For this review, take the finished solid that the model builds, in its own axes (mm). A direction names the side the tool comes from. Coordinates: 2 decimals unless noted, no trailing zeros. Loops run counter-clockwise (first coordinate to the right, second up) from the corner with the lowest first, then second, coordinate; pieces in that order, holes last. Notation, with made-up numbers: (78, 83) -> (83, 83) arc R25 ccw to (83, 101) -> close; hole circle Ø10 at (-38, 80). An arc over 180 degrees is marked (long way). Use a Markdown table: item, result.
from build123d import *

# Parameters (mm, degrees)
SKETCH1_W                           = 18.5
SKETCH1_H                           = 19.8
BE_00_BODY_DEPTH                    = 5.3
CE_00_MAIN_CAVITY_DEPTH             = 0.7112
CUT_EXTRUDE26_DEPTH                 = 1.5
CE_00_OUTPUT_CAVITY_DEPTH           = 2.75
CE_00_MULTIPIN_CAVITY_DEPTH         = 3.66
SKETCH43_W                          = 24.756879044
SKETCH43_H                          = 5.996687822
CE_00_NEAR_MULTIPIN_CONNECTOR_DEPTH = 2.75
CE_00_DC_BOARD_CAVITY_DEPTH         = 2
FILLET_A_0_4MM_R                    = 0.4
FILLET_B_0_2_R                      = 0.2
FILLET_C_0_16MM_R                   = 0.16
FILLET_E_0_05MM_R                   = 0.05
CHAMFER_A_0_10MM_SIZE               = 0.1
CHAMFER1_SIZE                       = 0.0508


# Read off the part's stored shape, not the designer's step: CSK for #0 Flat Head Machine Screw2
with BuildPart() as part:
    # Sketch1 → BE-00 Body (new body)
    with BuildSketch(Plane(origin=(0, 0, 0), x_dir=(1, 0, 0), z_dir=(0, 1, 0))):
        with Locations((0.75, 3.1)):
            Rectangle(SKETCH1_W, SKETCH1_H)
    extrude(amount=BE_00_BODY_DEPTH)

    # Sketch9 → CE-00 Main Cavity (cut)
    with BuildSketch(Plane(origin=(0, 0, 0), x_dir=(1, 0, 0), z_dir=(0, 1, 0))):
        with BuildLine():
            Line((2.146781775, -1.5534), (12.535922666, -1.5534))
            Line((12.535922666, -1.5534), (12.535922666, 2.0534))
            Line((12.535922666, 2.0534), (2.2, 2.0534))
            Line((2.2, 2.0534), (2.2, 6.384290248))
            Line((2.2, 6.384290248), (0, 6.384290248))
            Line((0, 6.384290248), (0, 2.4))
            Line((0, 2.4), (-10.40064316, 2.4))
            Line((-10.40064316, 2.4), (-10.40064316, -2.4))
            Line((-10.40064316, -2.4), (1, -2.4))
            ThreePointArc((1, -2.4), (1.712713126, -2.165422187), (2.146781775, -1.5534))
        make_face()
    extrude(amount=CE_00_MAIN_CAVITY_DEPTH, mode=Mode.SUBTRACT)

    # Sketch45 → Cut-Extrude26 (cut)
    with BuildSketch(Plane(origin=(0, 0, 0), x_dir=(1, 0, 0), z_dir=(0, 1, 0))):
        with BuildLine():
            Line((-0.5, -2.4), (-10.40064316, -2.4))
            Line((-10.40064316, -2.4), (-10.40064316, 2.4))
            Line((-10.40064316, 2.4), (-0.5, 2.4))
            ThreePointArc((-0.5, 2.4), (-0.075735931, 2.224264069), (0.1, 1.8))
            Line((0.1, 1.8), (0.1, -1.8))
            ThreePointArc((0.1, -1.8), (-0.075735931, -2.224264069), (-0.5, -2.4))
        make_face()
        with BuildLine():
            Line((12.535922666, -1.5534), (2.8, -1.5534))
            ThreePointArc((2.8, -1.5534), (2.375735931, -1.377664069), (2.2, -0.9534))
            Line((2.2, -0.9534), (2.2, 1.4534))
            ThreePointArc((2.2, 1.4534), (2.375735931, 1.877664069), (2.8, 2.0534))
            Line((2.8, 2.0534), (12.535922666, 2.0534))
            Line((12.535922666, 2.0534), (12.535922666, -1.5534))
        make_face()
    extrude(amount=CUT_EXTRUDE26_DEPTH, mode=Mode.SUBTRACT)

    # Sketch29 → CE-00 Output Cavity (cut)
    with BuildSketch(Plane.XZ):
        with BuildLine():
            Line((5.1994, -5.22), (5.1994, 10.160265554))
            Line((5.1994, 10.160265554), (12.409807772, 10.160265554))
            Line((12.409807772, 10.160265554), (12.409807772, -6.82))
            Line((12.409807772, -6.82), (6.7994, -6.82))
            ThreePointArc((6.7994, -6.82), (5.66802915, -6.35137085), (5.1994, -5.22))
        make_face()
    extrude(amount=-CE_00_OUTPUT_CAVITY_DEPTH, mode=Mode.SUBTRACT)

    # Sketch4 → CE-00 Multipin Cavity (cut)
    with BuildSketch(Plane(origin=(0, 0, 0), x_dir=(1, 0, 0), z_dir=(0, 1, 0))):
        with BuildLine():
            Line((-1.393549192, 5.214359354), (-3.1256, 6.214359354))
            ThreePointArc((-3.1256, 6.214359354), (-3.711240646, 6.8), (-3.9256, 7.6))
            Line((-3.9256, 7.6), (-3.9256, 16))
            Line((-3.9256, 16), (5.6756, 16))
            Line((5.6756, 16), (5.6756, 7.6))
            ThreePointArc((5.6756, 7.6), (5.461240646, 6.8), (4.8756, 6.214359354))
            Line((4.8756, 6.214359354), (3.143549192, 5.214359354))
            ThreePointArc((3.143549192, 5.214359354), (2.757659665, 5.054518678), (2.343549192, 5))
            Line((2.343549192, 5), (-0.593549192, 5))
            ThreePointArc((-0.593549192, 5), (-1.007659665, 5.054518678), (-1.393549192, 5.214359354))
        make_face()
    extrude(amount=CE_00_MULTIPIN_CAVITY_DEPTH, mode=Mode.SUBTRACT)

    # Sketch43 → CE-00 Near Multipin Connector (cut)
    with BuildSketch(Plane(origin=(0, 0, 0), x_dir=(1, 0, 0), z_dir=(0, 1, 0))):
        with Locations((0.495115422, 13.478343911)):
            Rectangle(SKETCH43_W, SKETCH43_H)
    extrude(amount=CE_00_NEAR_MULTIPIN_CONNECTOR_DEPTH, mode=Mode.SUBTRACT)

    # Sketch10 → CE-00 DC board Cavity (cut)
    with BuildSketch(Plane(origin=(0, 0, 0), x_dir=(1, 0, 0), z_dir=(0, 1, 0))):
        with BuildLine():
            Line((5.6756, 6.82), (5.6756, 7.6))
            Line((5.6756, 7.6), (-4.0752, 7.6))
            ThreePointArc((-4.0752, 7.6), (-4.499464069, 7.424264069), (-4.6752, 7))
            Line((-4.6752, 7), (-4.6752, 3.4))
            ThreePointArc((-4.6752, 3.4), (-4.499464069, 2.975735931), (-4.0752, 2.8))
            Line((-4.0752, 2.8), (8.306329243, 2.8))
            Line((8.306329243, 2.8), (8.306329243, 6.82))
            Line((8.306329243, 6.82), (5.6756, 6.82))
        make_face()
    extrude(amount=CE_00_DC_BOARD_CAVITY_DEPTH, mode=Mode.SUBTRACT)

    # CSK for #0 Flat Head Machine Screw2 outl → CSK for #0 Flat Head Machine Screw2 (revolve, cut)
    with BuildSketch(Plane(origin=(3, 0, 4.6), x_dir=(1, 0, 0), z_dir=(0, 0, 1))):
        Polygon((0, 0), (1.000000032, 0), (0.80645, 0.193550032), (0.80645, 4.489162828), (1.5113, 5.3), (0, 5.3), align=None)
    revolve(axis=Axis((3, 0, 4.6), (0, 1, 0)), mode=Mode.SUBTRACT)

    # CSK for _0 Flat Head Machine Screw2 2 ou → CSK for _0 Flat Head Machine Screw2 2 (revolve, cut)
    with BuildSketch(Plane(origin=(-1.5, 0, 4.6), x_dir=(1, 0, 0), z_dir=(0, 0, 1))):
        Polygon((0, 0), (1.000000032, 0), (0.80645, 0.193550032), (0.80645, 4.489162828), (1.5113, 5.3), (0, 5.3), align=None)
    revolve(axis=Axis((-1.5, 0, 4.6), (0, 1, 0)), mode=Mode.SUBTRACT)

    # CSK for _0 Flat Head Machine Screw2 3 ou → CSK for _0 Flat Head Machine Screw2 3 (revolve, cut)
    with BuildSketch(Plane(origin=(-6.3, 0, 4.6), x_dir=(1, 0, 0), z_dir=(0, 0, 1))):
        Polygon((0, 0), (1.000000032, 0), (0.80645, 0.193550032), (0.80645, 4.489162828), (1.5113, 5.3), (0, 5.3), align=None)
    revolve(axis=Axis((-6.3, 0, 4.6), (0, 1, 0)), mode=Mode.SUBTRACT)

    # CSK for _0 Flat Head Machine Screw2 4 ou → CSK for _0 Flat Head Machine Screw2 4 (revolve, cut)
    with BuildSketch(Plane(origin=(6.6, 0, 2.2), x_dir=(1, 0, 0), z_dir=(0, 0, 1))):
        Polygon((0, 2.75), (1.000000032, 2.75), (0.80645, 2.943550032), (0.80645, 4.489162828), (1.5113, 5.3), (0, 5.3), align=None)
    revolve(axis=Axis((6.6, 0, 2.2), (0, 1, 0)), mode=Mode.SUBTRACT)

    # CSK for _0 Flat Head Machine Screw2 5 ou → CSK for _0 Flat Head Machine Screw2 5 (revolve, cut)
    with BuildSketch(Plane(origin=(6.6, 0, -2.2), x_dir=(1, 0, 0), z_dir=(0, 0, 1))):
        Polygon((0, 2.75), (1.000000032, 2.75), (0.80645, 2.943550032), (0.80645, 4.489162828), (1.5113, 5.3), (0, 5.3), align=None)
    revolve(axis=Axis((6.6, 0, -2.2), (0, 1, 0)), mode=Mode.SUBTRACT)

    # CSK for _0 Flat Head Machine Screw2 6 ou → CSK for _0 Flat Head Machine Screw2 6 (revolve, cut)
    with BuildSketch(Plane(origin=(-6.3, 0, -4.6), x_dir=(1, 0, 0), z_dir=(0, 0, 1))):
        Polygon((0, 0), (1.000000032, 0), (0.80645, 0.193550032), (0.80645, 4.489162828), (1.5113, 5.3), (0, 5.3), align=None)
    revolve(axis=Axis((-6.3, 0, -4.6), (0, 1, 0)), mode=Mode.SUBTRACT)

    # CSK for _0 Flat Head Machine Screw2 7 ou → CSK for _0 Flat Head Machine Screw2 7 (revolve, cut)
    with BuildSketch(Plane(origin=(-6.3, 0, -8.7), x_dir=(1, 0, 0), z_dir=(0, 0, 1))):
        Polygon((0, 0), (1.000000032, 0), (0.80645, 0.193550032), (0.80645, 4.489162828), (1.5113, 5.3), (0, 5.3), align=None)
    revolve(axis=Axis((-6.3, 0, -8.7), (0, 1, 0)), mode=Mode.SUBTRACT)

    # CSK for _0 Flat Head Machine Screw2 8 ou → CSK for _0 Flat Head Machine Screw2 8 (revolve, cut)
    with BuildSketch(Plane(origin=(7.8, 0, -8.7), x_dir=(1, 0, 0), z_dir=(0, 0, 1))):
        Polygon((0, 0), (1.000000032, 0), (0.80645, 0.193550032), (0.80645, 4.489162828), (1.5113, 5.3), (0, 5.3), align=None)
    revolve(axis=Axis((7.8, 0, -8.7), (0, 1, 0)), mode=Mode.SUBTRACT)

    # Fillet A 0.4mm
    fillet_a_0_4mm_edges = [part.edges().sort_by_distance(p)[0] for p in [
        (10, 4.025, 6.8),
        (-8.5, 2.65, 6.8),
        (-8.5, 4.025, -13),
        (10, 4.025, -13),
    ]]
    fillet(fillet_a_0_4mm_edges, radius=FILLET_A_0_4MM_R)

    # Fillet B 0.2
    # the kernel refuses this fillet: 0.2 mm, written as the material it takes off along each edge
    with BuildSketch(Plane(origin=(5.6756, -0.5, -6.82), x_dir=(0, 0, -1), z_dir=(0, 1, 0))) as fillet_b_0_2_piece_1:
        with BuildLine():
            CenterArc((FILLET_B_0_2_R, -FILLET_B_0_2_R), FILLET_B_0_2_R, 90, 90)
            Line((0, -FILLET_B_0_2_R), (0, 0))
            Line((0, 0), (FILLET_B_0_2_R, 0))
        make_face()
    extrude(amount=2.5, mode=Mode.SUBTRACT)
    with BuildSketch(Plane(origin=(5.6756, -0.5, -10.48), x_dir=(0, 0, 1), z_dir=(0, 1, 0)), Plane(origin=(-3.9256, 2.75, -10.48), x_dir=(0, 0, 1), z_dir=(0, -1, 0))) as fillet_b_0_2_piece_2:
        with BuildLine():
            CenterArc((FILLET_B_0_2_R, FILLET_B_0_2_R), FILLET_B_0_2_R, 180, 90)
            Line((0, FILLET_B_0_2_R), (0, 0))
            Line((0, 0), (FILLET_B_0_2_R, 0))
        make_face()
    extrude(amount=3.25, mode=Mode.SUBTRACT)
    with BuildSketch(Plane(origin=(-3.9256, -0.496027054, -7.6), x_dir=(0, 0, -1), z_dir=(0, 1, 0))) as fillet_b_0_2_piece_3:
        with BuildLine():
            CenterArc((0.198410822, 0.2), FILLET_B_0_2_R, 183.612026157, 86.387973843)
            Line((-0.001191884, 0.1874), (-0.021152154, 0.18614))
            ThreePointArc((-0.021152154, 0.18614), (-0.02, 0.1496), (-0.02, 0))
            Line((-0.02, 0), (0, -0.02))
            Line((0, -0.02), (0.198410822, -0.02))
            Line((0.198410822, -0.02), (0.198410822, 0))
        make_face()
    extrude(amount=2.496027054, mode=Mode.SUBTRACT)

    # Fillet C 0.16mm
    fillet_c_0_16mm_edges = [part.edges().sort_by_distance(p)[0] for p in [
        (2.2, 0.3556, -2.8),
        (0, 0.3556, -2.8),
        (0, 0.3556, -2.4),
        (2.146781775, 0.3556, 1.5534),
        (2.2, 0.3556, -2.0534),
    ]]
    fillet(fillet_c_0_16mm_edges, radius=FILLET_C_0_16MM_R)

    # Fillet E 0.05mm
    fillet_e_0_05mm_edges = [part.edges().sort_by_distance(p)[0] for p in [
        (5.1994, 0.75, 1.5534),
        (5.1994, 0.75, -2.0534),
        (5.1994, 1, -2.8),
    ]]
    fillet(fillet_e_0_05mm_edges, radius=FILLET_E_0_05MM_R)

    # Chamfer A 0.10mm
    chamfer_a_0_10mm_edges = [part.edges().sort_by_distance(p)[0] for p in [
        (-8.5, 5.3, -3.1),
        (0.75, 5.3, -13),
        (10, 5.3, -3.1),
        (0.75, 5.3, 6.8),
        (-8.382842712, 5.3, 6.682842712),
        (9.882842712, 5.3, 6.682842712),
        (9.882842712, 5.3, -12.882842712),
        (-8.382842712, 5.3, -12.882842712),
    ]]
    chamfer(chamfer_a_0_10mm_edges, length=CHAMFER_A_0_10MM_SIZE)

    # Chamfer1
    chamfer1_edges = [part.edges().sort_by_distance(p)[0] for p in [
        (10, 1.375, -6.82),
        (5.1994, 1.375, 6.8),
        (5.6756, 3.205, -13),
        (-3.9256, 3.205, -13),
        (10, 1.375, -10.48),
        (-8.5, 1.375, -10.48),
        (-8.5, 0.75, -2.4),
        (-8.5, 0.75, 2.4),
    ]]
    chamfer(chamfer1_edges, length=CHAMFER1_SIZE)


solid = part.part
(1) Take a section at A-A on z = -4.6. Write out the cut boundary in (x, y), plus the area to 3 significant figures.
Found:
| item | result |
|---|---|
| outline | (-8.5, 0) -> (-7.3, 0) -> (-7.11, 0.19) -> (-7.11, 4.49) -> (-7.81, 5.3) -> (-8.4, 5.3) -> (-8.5, 5.2) -> close; (-5.49, 0.19) -> (-5.3, 0) -> (-4.68, 0) -> (-4.68, 2) -> (5.2, 2) -> (5.2, 2.75) -> (10, 2.75) -> (10, 5.2) -> (9.9, 5.3) -> (-4.79, 5.3) -> (-5.49, 4.49) -> close |
| area | 55.9 mm^2 |
(2) For line 1 along Z through (x, y) = (-6.3, 2.3); line 2 along X through (y, z) = (3.05, 4.6); line 3 along Z through (x, y) = (-6.3, 1.35), list the stretches that pass through material, from the lowest coordinate up.
Found:
| item | result |
|---|---|
| line 1 | z = -10.48 to -9.51, -7.89 to -5.41, -3.79 to 3.79, 5.41 to 6.8 |
| line 2 | x = -8.5 to -7.11, -5.49 to -2.31, -0.69 to 2.19, 3.81 to 10 |
| line 3 | z = -10.48 to -9.51, -7.89 to -5.41, -3.79 to -2.4, 2.4 to 3.79, 5.41 to 6.8 |
(3) For pin 1 Ø2 at (x, z) = (9, -12) entering from -Y; pin 2 Ø1.8 at (x, y) = (0.5, 2.5) entering from -Z; pin 3 Ø2 at (x, z) = (6.6, 2.2) entering from +Y, all flat-tipped, find the tip position at first contact; note any pin that passes through.
Found:
| item | result |
|---|---|
| pin 1 | stops at y = 2.75 |
| pin 2 | stops at z = -5 |
| pin 3 | stops at y = 4.71 |
(4) For faces 4 (the face through (4, 1.5, 0)), 5 (the face through (0, 0, 5)), 6 (the face through (5.199, 2, 2)), 7 (the face through (-6.4, 2.4, -5.4)), 8 (the face through (1, 3.66, -9)), list the 3-axis set-ups (+Z, -Z, +X, -X, +Y, -Y) from which the entire face can be reached by the end or side of a thin tool; tool diameter is ignored.
Found:
| item | result |
|---|---|
| face 4 | +X, -Y |
| face 5 | +Z, -Z, +X, -X, -Y |
| face 6 | +Z, +X, -Y |
| face 7 | +Y, -Y |
| face 8 | -Z, -Y |
(5) Mouldability with a two-part tool opening along Z and no side actions: class faces 1 (the face through (-3.705, 2.818, -6.79)), 2 (the face through (-4.675, 1, -5)), 3 (the face through (-3.926, 2, -10)) as pulls with the +Z half, pulls with the -Z half, needs draft (parallel to the pull), parting line crosses it, or undercut.
Found:
| item | result |
|---|---|
| face 1 | pulls with the -Z half |
| face 2 | undercut |
| face 3 | needs draft |
(6) Take a section at B-B on y = 4.2. State how many separate pieces and enclosed holes the cut face has, plus the area to 3 significant figures.
Found:
| item | result |
|---|---|
| separate pieces | 1 |
| enclosed holes | 8 |
| area | 350 mm^2 |
